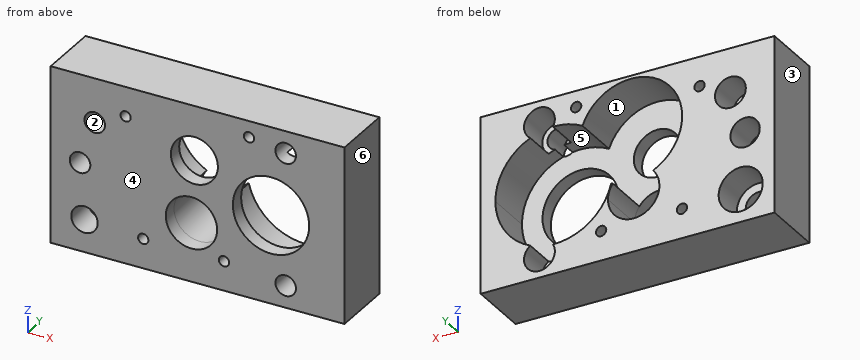
from build123d import *
from build123d.topology import SkipClean

# Parameters (mm, degrees)
SKETCH_1_W          = 20
SKETCH_1_H          = 12
SKETCH_1_R          = 1.75
SKETCH_1_R_2        = 1.6
SKETCH_1_R_3        = 2.6
EXTRUDE_1_DEPTH     = 1
EXTRUDE_START       = 1
SKETCH_1_6_W        = 20
SKETCH_1_6_H        = 12
EXTRUDE_2_DEPTH     = 3.2
SKETCH_4_R          = 0.9
SKETCH_4_R_2        = 0.35
SKETCH_4_R_3        = 0.7
CUT_EXTRUDE_1_DEPTH = 24.698945124
SKETCH_4_3_R        = 1.5
SKETCH_4_3_R_2      = 1
SKETCH_4_3_R_3      = 1.05
CUT_EXTRUDE_4_DEPTH = 2.2


with BuildPart() as part:
    # 草图1 → 凸台-拉伸1 (new body)
    with BuildSketch(Plane(origin=(0, 0, 0), x_dir=(1, 0, 0), z_dir=(0, 1, 0))):
        with Locations((10, -6)):
            Rectangle(SKETCH_1_W, SKETCH_1_H)
        with Locations(Location((9.582575695, -4, 0), (0, 0, 270))):
            Circle(SKETCH_1_R, mode=Mode.SUBTRACT)
        with Locations(Location((9.782588007, -8.295345746, 0), (0, 0, 270))):
            Circle(SKETCH_1_R_2, mode=Mode.SUBTRACT)
        with Locations(Location((15, -6, 0), (0, 0, 270))):
            Circle(SKETCH_1_R_3, mode=Mode.SUBTRACT)
    extrude(amount=EXTRUDE_1_DEPTH)

    # 草图1<6> → 凸台-拉伸2 (add)
    with SkipClean():  # the faces are left unmerged after this step: merging them gives an invalid solid
        with BuildSketch(Plane(origin=(0, 0, 0), x_dir=(1, 0, 0), z_dir=(0, 1, 0)).offset(EXTRUDE_START)):
            with Locations((10, -6)):
                Rectangle(SKETCH_1_6_W, SKETCH_1_6_H)
            with BuildLine():
                ThreePointArc((8.258713369, -5.144503622), (8.971944493, -2.359990995), (11.332575695, -4))
                ThreePointArc((11.332575695, -4), (11.249212779, -4.53368608), (11.007066173, -5.01652687))
                ThreePointArc((11.007066173, -5.01652687), (11.059967321, -5.036772118), (11.112533909, -5.05787082))
                ThreePointArc((11.112533909, -5.05787082), (15.47441313, -2.028233116), (19, -6))
                ThreePointArc((19, -6), (17.033646838, -9.444456494), (13.067859731, -9.502404029))
                ThreePointArc((13.067859731, -9.502404029), (7.432385055, -10.888904322), (8.258713369, -5.144503622))
            make_face(mode=Mode.SUBTRACT)
        extrude(amount=EXTRUDE_2_DEPTH)

    # 草图4 → 切除-拉伸1 (cut, through all)
    with SkipClean():  # the faces are left unmerged after this step: merging them gives an invalid solid
        with BuildSketch(Plane(origin=(0, 4.2, 0), x_dir=(1, 0, 0), z_dir=(0, 1, 0))):
            with Locations(Location((2.3, -2.214171161, 0), (0, 0, 270))):
                Circle(SKETCH_4_R)
            with Locations(Location((6.3, -2, 0), (0, 0, 270))):
                Circle(SKETCH_4_R_2)
            with Locations(Location((5.1, -10, 0), (0, 0, 270))):
                Circle(SKETCH_4_R_2)
            with Locations(Location((11.8, -2, 0), (0, 0, 270))):
                Circle(SKETCH_4_R_2)
            with Locations(Location((2, -6, 0), (0, 0, 270))):
                Circle(SKETCH_4_R_3)
            with Locations(Location((16, -1.5, 0), (0, 0, 270))):
                Circle(SKETCH_4_R_3)
            with Locations(Location((16, -10.5, 0), (0, 0, 270))):
                Circle(SKETCH_4_R_3)
            with Locations(Location((3, -9, 0), (0, 0, 270))):
                Circle(SKETCH_4_R_3)
            with Locations(Location((13.5, -10.9, 0), (0, 0, 270))):
                Circle(SKETCH_4_R_2)
        extrude(amount=-CUT_EXTRUDE_1_DEPTH, mode=Mode.SUBTRACT)

    # 草图4<3> → 切除-拉伸4 (cut)
    with SkipClean():  # the faces are left unmerged after this step: merging them gives an invalid solid
        with BuildSketch(Plane(origin=(0, 4.2, 0), x_dir=(1, 0, 0), z_dir=(0, 1, 0))):
            with Locations(Location((2.3, -2.214171161, 0), (0, 0, 270))):
                Circle(SKETCH_4_3_R)
            with Locations(Location((2, -6, 0), (0, 0, 270))):
                Circle(SKETCH_4_3_R_2)
            with Locations((16, -1.5)):
                Circle(SKETCH_4_3_R_3)
            with Locations((16, -10.5)):
                Circle(SKETCH_4_3_R_3)
            with Locations(Location((3, -9, 0), (0, 0, 270))):
                Circle(SKETCH_4_3_R_3)
        extrude(amount=-CUT_EXTRUDE_4_DEPTH, mode=Mode.SUBTRACT)


solid = part.part
Read the model definition and answer for the solid it produces. Units are mm, in the model's axes. Face numbers are marked on the shaded views. A direction names the side the tool comes from. Give positions to 0.01 mm unless a question says otherwise; leave off trailing zeros. Loops run counter-clockwise (first coordinate to the right, second up) from the corner with the lowest first, then second, coordinate; pieces in that order, holes last. Notation, with made-up numbers: M 75.25,-27 L 130.25,-27 A12 cw 130.25,-23 Z; hole C 27.25,-6 d9. An arc over 180 degrees is marked long. Write each question's results on one line, items separated by ' | '.
1. Section D-D on z = 10.9 is taken. Give the vertices of the cut face in (x, y).
Values:
outline: M 0,0 L 13.15,0 L 13.15,4.2 L 12.12,4.2 L 12.12,1 L 7.44,1 L 7.44,4.2 L 0,4.2 Z; M 13.85,0 L 15.43,0 L 15.43,2 L 15.03,2 L 15.03,4.2 L 13.85,4.2 Z; M 16.57,0 L 20,0 L 20,4.2 L 16.97,4.2 L 16.97,2 L 16.57,2 Z
2. Straight lines are drawn through the part: line 1 (X direction, y = 1.1, z = 11); line 2 (Z direction, x = 16, y = 3.05); line 3 (X direction, y = 3.5, z = 1.5). For each, find the intervals that lie inside material, in ascending order. Write a range as [from, to].
Values:
line 1: x = [0, 7.56], [12, 13.16], [13.84, 15.51], [16.49, 20] | line 2: z = [0, 0.45], [11.55, 12] | line 3: x = [0, 0.98], [3.62, 14.95], [17.05, 20]
3. A tool of negligible diameter and unlimited length cuts with its end or side. For the marked faces 1 and 2, from which of +Z, -Z, +X, -X, +Y, -Y can it reach the whole face along a straight path? Write none if from no direction.
Values:
face 1: +Y | face 2: +Y, -Y
4. Given pin 1 (1.5 mm diameter, centred on x = 1.5, z = 2, fed in from +Y); pin 2 (2 mm diameter, centred on x = 9.58, z = 4, fed in from -Y), each flat-ended and moving along its own axis, determine where each tip first touches the part or whether it passes through.
Values:
pin 1: stops at y = 4.2 | pin 2: passes through
5. Section A-A on z = 9 is taken. Give the vertices of the cut face in (x, y), plus the area to 3 significant figures.
Values:
outline: M 0,0 L 2.3,0 L 2.3,2 L 1.95,2 L 1.95,4.2 L 0,4.2 Z; M 3.7,0 L 8.35,0 L 8.35,1 L 6.35,1 L 6.35,4.2 L 4.05,4.2 L 4.05,2 L 3.7,2 Z; M 11.22,0 L 20,0 L 20,4.2 L 17.65,4.2 L 17.65,1 L 11.22,1 Z | area: 37.6 mm^2
6. Section C-C on y = 2.9 is taken. State how many separate pieces and enclosed holes the cut face has, plus the area to 3 significant figures.
Values:
separate pieces: 1 | enclosed holes: 8 | area: 128 mm^2
7. The mould has two halves that part along X. Classify the marked faces 3, 4, 5 and 6: pulls with the +X half, pulls with the -X half, needs draft (parallel to the pull), parting line crosses it, or undercut.
Values:
face 3: pulls with the -X half | face 4: needs draft | face 5: undercut | face 6: pulls with the +X half
8. Section B-B on x = 11.8 is taken. Give the vertices of the cut face in (y, z).
Values:
outline: M 0,0 L 4.2,0 L 4.2,1.65 L 0,1.65 Z; M 0,2.35 L 4.2,2.35 L 4.2,3.6 L 1,3.6 L 1,11.16 L 4.2,11.16 L 4.2,12 L 0,12 Z
